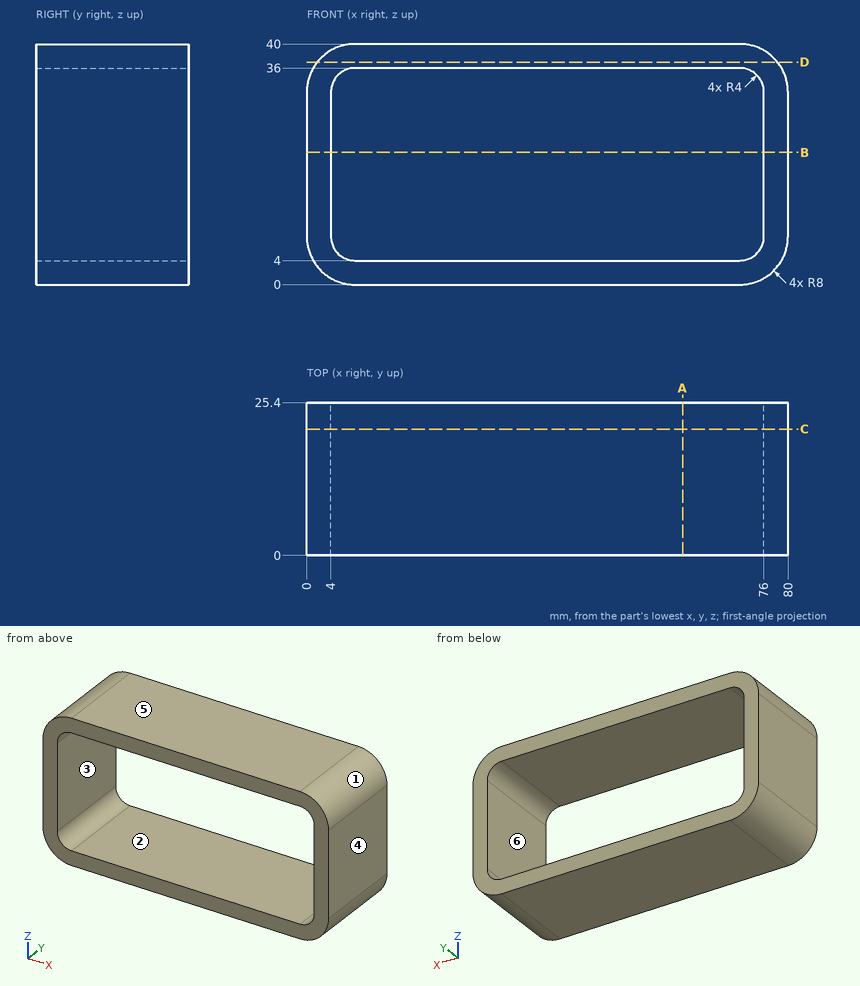
Here's the drawing with two shaded views (mm, measured from the low corner). I have some questions. A direction names the side the tool comes from. Coordinates: 2 decimals unless noted, no trailing zeros. Order: outer loops, then holes, each group sorted by start corner. A loop starts at its lowest first (then second) coordinate and runs counter-clockwise, first axis right, second up. Notation, with made-up numbers: M -32,48.5 L 0,48.5 A8 ccw 0,56.5 Z; hole C -17,67 d11. An arc over 180 degrees is marked long. Write item = value, one per line.
(1) If we mould it in two halves opening along X, with no side actions, what happens to the marked faces 3, 4, 5 and 6? For each: pulls with the +X half, pulls with the -X half, needs draft (parallel to the pull), parting line crosses it, or undercut.
Results are:
face_3 = undercut
face_4 = pulls with the +X half
face_5 = needs draft
face_6 = undercut
(2) For the marked faces 1 and 2, which set-ups out of +Z, -Z, +X, -X, +Y, -Y let a thin tool reach every point of the face, with its end or its side?
Results are:
face_1 = +Z, +X, +Y, -Y
face_2 = +Y, -Y
(3) Suppose I cut it at C-C on y = 21. Please give me the cut outline in (x, z), plus the area to 3 significant figures.
Results are:
outline = M 0,8 A8 ccw 8,0 L 72,0 A8 ccw 80,8 L 80,32 A8 ccw 72,40 L 8,40 A8 ccw 0,32 Z; hole M 4,8 A4 ccw 8,4 L 72,4 A4 ccw 76,8 L 76,32 A4 ccw 72,36 L 8,36 A4 ccw 4,32 Z
area = 855 mm2
(4) I need wall thicknesses on line 1 along X through (y, z) = (4.5, 18.5); line 2 along Z through (x, y) = (23, 17.75); line 3 along X through (y, z) = (8, 5). Which ranges of each line are inside material? Lowest first, please. Write a range as [from, to].
Results are:
line_1 = [0, 4], [76, 80]
line_2 = [0, 4], [36, 40]
line_3 = [0.58, 5.35], [74.65, 79.42]
(5) Suppose I cut it at D-D on z = 37. Please give me the cut outline in (x, y) (3 decimals).
Results are:
outline = M 1.755,0 L 78.245,0 L 78.245,25.4 L 1.755,25.4 Z
(6) Suppose I cut it at A-A on x = 62.5. Please give me the cut outline in (y, z).
Results are:
outline = M 0,0 L 25.4,0 L 25.4,4 L 0,4 Z; M 0,36 L 25.4,36 L 25.4,40 L 0,40 Z
(7) Suppose I cut it at B-B on z = 22. Please give me the cut outline in (x, y).
Results are:
outline = M 0,0 L 4,0 L 4,25.4 L 0,25.4 Z; M 76,0 L 80,0 L 80,25.4 L 76,25.4 Z
